For this review, take the finished solid that the model builds, in its own axes (mm). Round coordinates to 2 decimals unless told otherwise and drop trailing zeros. Write each loop counter-clockwise with the first axis right and the second up, starting at its lowest first coordinate (ties: lowest second). Pieces come first, ordered by that corner, then holes. Notation, with made-up numbers: M 42.25,-14 L 66.25,-14 A28 ccw 66.25,6 Z; hole C 82.25,19.5 d3. An arc over 180 degrees is marked long. Answer in a Markdown table with one row per item.
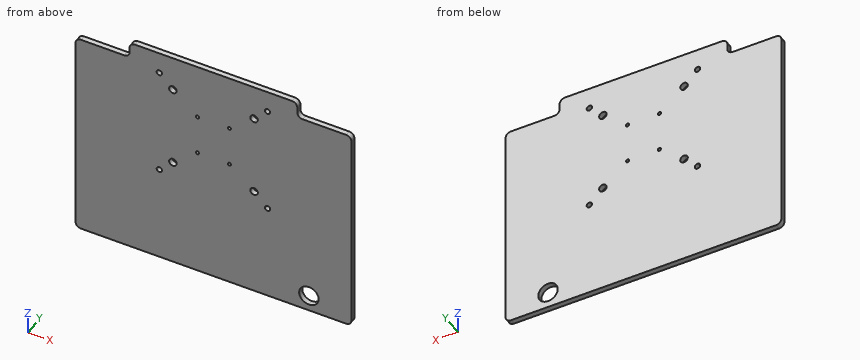
```python
from build123d import *

# Parameters (mm, degrees)
F1_DEPTH = 5


with BuildPart() as f1:
    # F0 (on Front) → F1 (new body)
    with BuildSketch(Plane.XZ):
        with BuildLine():
            Line((88.225863874, -105), (122.5, -105))
            ThreePointArc((122.5, -105), (126.0355339059, -103.5355339059), (127.5, -100))
            Line((127.5, -100), (127.5, 85))
            ThreePointArc((127.5, 85), (126.0355339059, 88.5355339059), (122.5, 90))
            Line((122.5, 90), (82.5, 90))
            ThreePointArc((82.5, 90), (78.9644660941, 91.4644660941), (77.5, 95))
            Line((77.5, 95), (77.5, 100))
            ThreePointArc((77.5, 100), (76.0355339059, 103.5355339059), (72.5, 105))
            Line((72.5, 105), (0, 105))
            Line((0, 105), (-72.5, 105))
            ThreePointArc((-72.5, 105), (-76.0355339059, 103.5355339059), (-77.5, 100))
            Line((-77.5, 100), (-77.5, 95))
            ThreePointArc((-77.5, 95), (-78.9644660941, 91.4644660941), (-82.5, 90))
            Line((-82.5, 90), (-122.5, 90))
            ThreePointArc((-122.5, 90), (-126.0355339059, 88.5355339059), (-127.5, 85))
            Line((-127.5, 85), (-127.5, -100))
            ThreePointArc((-127.5, -100), (-126.0355339059, -103.5355339059), (-122.5, -105))
            Line((-122.5, -105), (88.225863874, -105))
        make_face()
        with BuildLine():
            ThreePointArc((97.225863874, -90), (94.5898249046, -96.3639610307), (88.225863874, -99))
            ThreePointArc((88.225863874, -99), (81.8619028433, -83.6360389693), (97.225863874, -90))
        make_face(mode=Mode.SUBTRACT)
        with BuildLine():
            Line((-47.5, 85), (0, 85))
            Line((0, 85), (47.5, 85))
            ThreePointArc((47.5, 85), (50, 87.5), (52.5, 85))
            ThreePointArc((52.5, 85), (51.767766953, 83.232233047), (50, 82.5))
            Line((50, 82.5), (50, -12.5))
            ThreePointArc((50, -12.5), (51.767766953, -13.232233047), (52.5, -15))
            ThreePointArc((52.5, -15), (50, -17.5), (47.5, -15))
            Line((47.5, -15), (-47.5, -15))
            ThreePointArc((-47.5, -15), (-51.767766953, -16.767766953), (-50, -12.5))
            Line((-50, -12.5), (-50, 82.5))
            ThreePointArc((-50, 82.5), (-51.767766953, 86.767766953), (-47.5, 85))
        make_face(mode=Mode.SUBTRACT)
        with BuildLine():
            Line((47.5, 85), (0, 85))
            Line((0, 85), (-47.5, 85))
            ThreePointArc((-47.5, 85), (-48.232233047, 83.232233047), (-50, 82.5))
            Line((-50, 82.5), (-50, -12.5))
            ThreePointArc((-50, -12.5), (-48.232233047, -13.232233047), (-47.5, -15))
            Line((-47.5, -15), (47.5, -15))
            ThreePointArc((47.5, -15), (48.232233047, -13.232233047), (50, -12.5))
            Line((50, -12.5), (50, 82.5))
            ThreePointArc((50, 82.5), (48.232233047, 83.232233047), (47.5, 85))
        make_face()
        with BuildLine():
            Line((34, -2.5), (-34, -2.5))
            ThreePointArc((-34, -2.5), (-39.9748737342, -4.9748737342), (-37.5, 1))
            Line((-37.5, 1), (-37.5, 69))
            ThreePointArc((-37.5, 69), (-39.9748737342, 74.9748737342), (-34, 72.5))
            Line((-34, 72.5), (34, 72.5))
            ThreePointArc((34, 72.5), (37.5, 76), (41, 72.5))
            ThreePointArc((41, 72.5), (39.9748737342, 70.0251262658), (37.5, 69))
            Line((37.5, 69), (37.5, 1))
            ThreePointArc((37.5, 1), (39.9748737342, -0.0251262658), (41, -2.5))
            ThreePointArc((41, -2.5), (37.5, -6), (34, -2.5))
        make_face(mode=Mode.SUBTRACT)
        with BuildLine():
            ThreePointArc((-37.5, 1), (-35.0251262658, -0.0251262658), (-34, -2.5))
            Line((-34, -2.5), (34, -2.5))
            ThreePointArc((34, -2.5), (35.0251262658, -0.0251262658), (37.5, 1))
            Line((37.5, 1), (37.5, 69))
            ThreePointArc((37.5, 69), (35.0251262658, 70.0251262658), (34, 72.5))
            Line((34, 72.5), (-34, 72.5))
            ThreePointArc((-34, 72.5), (-35.0251262658, 70.0251262658), (-37.5, 69))
            Line((-37.5, 69), (-37.5, 1))
        make_face()
        with BuildLine():
            Line((13.25, 16.5), (-13.25, 16.5))
            ThreePointArc((-13.25, 16.5), (-15.8106601718, 15.4393398282), (-14.75, 18))
            Line((-14.75, 18), (-14.75, 52))
            ThreePointArc((-14.75, 52), (-15.8106601718, 54.5606601718), (-13.25, 53.5))
            Line((-13.25, 53.5), (13.25, 53.5))
            ThreePointArc((13.25, 53.5), (14.75, 55), (16.25, 53.5))
            ThreePointArc((16.25, 53.5), (15.8106601718, 52.4393398282), (14.75, 52))
            Line((14.75, 52), (14.75, 18))
            ThreePointArc((14.75, 18), (15.8106601718, 17.5606601718), (16.25, 16.5))
            ThreePointArc((16.25, 16.5), (14.75, 15), (13.25, 16.5))
        make_face(mode=Mode.SUBTRACT)
        with BuildLine():
            ThreePointArc((-14.75, 18), (-13.6893398282, 17.5606601718), (-13.25, 16.5))
            Line((-13.25, 16.5), (13.25, 16.5))
            ThreePointArc((13.25, 16.5), (13.6893398282, 17.5606601718), (14.75, 18))
            Line((14.75, 18), (14.75, 52))
            ThreePointArc((14.75, 52), (13.6893398282, 52.4393398282), (13.25, 53.5))
            Line((13.25, 53.5), (-13.25, 53.5))
            ThreePointArc((-13.25, 53.5), (-13.6893398282, 52.4393398282), (-14.75, 52))
            Line((-14.75, 52), (-14.75, 18))
        make_face()
    extrude(amount=F1_DEPTH)


solid = f1.part
```
Q1. Take a section at A-A (x = 108.5). State the section outline as (y, z) points, then the cut area to 3 significant figures.
Found:
| item | result |
|---|---|
| outline | M -5,-105 L 0,-105 L 0,90 L -5,90 Z |
| area | 975 mm² |
Q2. Take a section at B-B (y = -4). State how many separate pieces and enclosed holes the cut face has, then the cut area to 3 significant figures.
Found:
| item | result |
|---|---|
| separate pieces | 1 |
| enclosed holes | 13 |
| area | 51,500 mm² |
Q3. For probe 1 along X at (y, z) = (-3.9, 16.5); probe 2 along X at (y, z) = (-2.6, 85); probe 3 along Z at (x, y) = (-37.5, -1.65), list the stretches that pass through material, from the lowest coordinate up.
Found:
| item | result |
|---|---|
| probe 1 | -127.5 to -16.25, -13.25 to 13.25, 16.25 to 127.5 |
| probe 2 | -127.5 to -52.5, -47.5 to 47.5, 52.5 to 127.5 |
| probe 3 | -105 to -6, 1 to 69, 76 to 105 |
Q4. Insertion check: P1, Ø1.5, axis at x = 109.5, y = -3.5, coming from the +Z side; P2, Ø14.5, axis at x = 88.23, z = -90, coming from the +Y side; P3, Ø1.5, axis at y = -2.5, z = 97, coming from the -X side. Each pin has a flat end and moves straight along its axis. Give the tip position at first contact, or say it passes through.
Found:
| item | result |
|---|---|
| P1 | z = 90 |
| P2 | through |
| P3 | x = -77.5 |
